The model under review builds one solid part; all positions refer to its coordinate system, in mm. A direction names the side the tool comes from. Coordinates: 2 decimals unless noted, no trailing zeros. Order: outer loops, then holes, each group sorted by start corner. A loop starts at its lowest first (then second) coordinate and runs counter-clockwise, first axis right, second up.
```python
from build123d import *

# Parameters (mm, degrees)
SKETCH1_R                = 71
SKETCH1_R_2              = 50
BOSS_EXTRUDE1_DEPTH      = 44
SKETCH2_R                = 24.216288289
SKETCH2_R_2              = 19.150259362
BOSS_EXTRUDE2_DEPTH      = 54
BOSS_EXTRUDE2_DEPTH_BACK = 10
SKETCH3_R                = 19.150259362
BOSS_EXTRUDE3_DEPTH      = 30
SKETCH4_R                = 19.150259362
BOSS_EXTRUDE4_DEPTH      = 74
SKETCH7_R                = 50
BOSS_EXTRUDE5_DEPTH      = 1
BOSS_EXTRUDE5_DEPTH_BACK = 44


with BuildPart() as part:
    # Sketch1 → Boss-Extrude1 (new body)
    with BuildSketch(Plane.XY):
        Circle(SKETCH1_R)
        Circle(SKETCH1_R_2, mode=Mode.SUBTRACT)
    extrude(amount=BOSS_EXTRUDE1_DEPTH)



with BuildPart() as body_2:
    # Sketch2 → Boss-Extrude2 (new body, two sides)
    with BuildSketch(Plane.XY) as boss_extrude2_sk:
        Circle(SKETCH2_R)
        Circle(SKETCH2_R_2, mode=Mode.SUBTRACT)
    extrude(amount=BOSS_EXTRUDE2_DEPTH)
    extrude(boss_extrude2_sk.sketch, amount=-BOSS_EXTRUDE2_DEPTH_BACK)


with BuildPart() as body_3:
    # Sketch3 → Boss-Extrude3 (new body)
    with BuildSketch(Plane.XY):
        Circle(SKETCH3_R)
    extrude(amount=-BOSS_EXTRUDE3_DEPTH)


with BuildPart() as body_4:
    # Sketch4 → Boss-Extrude4 (new body)
    with BuildSketch(Plane.XY):
        Circle(SKETCH4_R)
    extrude(amount=BOSS_EXTRUDE4_DEPTH)


with BuildPart() as part_1:
    add(part.part)

    add(body_2.part)  # Boss-Extrude5 merges body 2

    add(body_3.part)  # Boss-Extrude5 merges body 3

    add(body_4.part)  # Boss-Extrude5 merges body 4
    # Sketch7 → Boss-Extrude5 (add, two sides)
    with BuildSketch(Plane.XY.offset(44)) as boss_extrude5_sk:
        Circle(SKETCH7_R)
    extrude(amount=BOSS_EXTRUDE5_DEPTH)
    extrude(boss_extrude5_sk.sketch, amount=-BOSS_EXTRUDE5_DEPTH_BACK)


solid = part_1.part
```
(1) We need section D-D, the plane x = -28. Write out the cut boundary in (y, z).
A:
outline: (-65.25, 0) - (65.25, 0) - (65.25, 44) - (41.42, 44) - (41.42, 45) - (-41.42, 45) - (-41.42, 44) - (-65.25, 44) - close
(2) Wall thickness on probe 1 along Z at (x, y) = (22.5, 48); probe 2 along Z at (x, y) = (35, -32); probe 3 along Y at (x, z) = (-36, 21): over which ranges is each line inside the solid? List them lowest first.
A:
probe 1: z = 0 to 44
probe 2: z = 0 to 45
probe 3: y = -61.2 to 61.2
(3) Machinability: for faces 1 (the face through (18, 7, -10)), 2 (the face through (18, 7, 54)), 3 (the face through (0, 0, -30)), which of the approach directions +Z, -Z, +X, -X, +Y, -Y give a long, thin tool a straight path to every point of the face, cutting with its end or side? Answer none if there is none.
A:
face 1: -Z
face 2: +Z
face 3: -Z, +X, -X, +Y, -Y
(4) We need section A-A, the plane x = 0. Write out the cut boundary in (y, z).
A:
outline: (-71, 0) - (-24.22, 0) - (-24.22, -10) - (-19.15, -10) - (-19.15, -30) - (19.15, -30) - (19.15, -10) - (24.22, -10) - (24.22, 0) - (71, 0) - (71, 44) - (50, 44) - (50, 45) - (24.22, 45) - (24.22, 54) - (19.15, 54) - (19.15, 74) - (-19.15, 74) - (-19.15, 54) - (-24.22, 54) - (-24.22, 45) - (-50, 45) - (-50, 44) - (-71, 44) - close
(5) For pin 1 Ø6 at (x, z) = (30.5, 34.5) entering from -Y; pin 2 Ø8 at (y, z) = (-49.5, 39.5) entering from -X; pin 3 Ø2 at (y, z) = (38.5, -1.5) entering from +X; pin 4 Ø8 at (y, z) = (30.5, 10.5) entering from +X, all flat-tipped, find the tip position at first contact; note any pin that passes through.
A:
pin 1: stops at y = -65.46
pin 2: stops at x = -54.5
pin 3: passes through
pin 4: stops at x = 65.87
(6) We need section C-C, the plane z = 56. Write out the cut boundary in (x, y), and give its area (3 significant figures).
A:
outline: circle Ø38.3 at (0, 0)
area: 1,150 mm2
